```python
from build123d import *

# Parameters (mm, degrees)
SKETCH1_R           = 2
BOSS_EXTRUDE1_DEPTH = 89
SKETCH2_R           = 3
BOSS_EXTRUDE2_DEPTH = 2
CHAMFER1_SIZE       = 1


with BuildPart() as part:
    # Sketch1 → Boss-Extrude1 (new body)
    with BuildSketch(Plane(origin=(0, 0, 0), x_dir=(1, 0, 0), z_dir=(0, 1, 0))):
        with Locations(Location((0, 0, 0), (0, 0, 270))):
            Circle(SKETCH1_R)
    extrude(amount=BOSS_EXTRUDE1_DEPTH)

    # Sketch2 → Boss-Extrude2 (add)
    with BuildSketch(Plane.XZ):
        with Locations(Location((0, 0, 0), (0, 0, 270))):
            Circle(SKETCH2_R)
    extrude(amount=BOSS_EXTRUDE2_DEPTH)

    # Chamfer1
    chamfer1_edges = [part.edges().sort_by_distance(p)[0] for p in [
        (0, -2, 3),
    ]]
    chamfer(chamfer1_edges, length=CHAMFER1_SIZE)


solid = part.part
```
Check sheet for the modelled part. Datum: model origin and axes. Units: mm. A direction names the side the tool comes from. Give positions to 0.01 mm unless a question says otherwise; leave off trailing zeros. Write each loop counter-clockwise with the first axis right and the second up, starting at its lowest first coordinate (ties: lowest second). Pieces come first, ordered by that corner, then holes.
Item 1: Scan lines: L1, parallel to Z at x = 0.2, y = 62.5; L2, parallel to X at y = 50, z = 0; L3, parallel to Z at x = 0.65, y = 81. Record each from-to range of solid material in increasing order.
Item 2: Gauge pin test, flat ends, axial feed: pin 1 (2 mm diameter, centred on x = 2, y = 35, fed in from -Z); pin 2 (3 mm diameter, centred on y = 29.5, z = 0, fed in from +X). Record the tip position at first contact, or that the pin passes through.
Item 3: Access from +Z, -Z, +X, -X, +Y, -Y to the whole of each face (thin tool, end or side, straight path). Record for faces 1 (the face through (-1, 0, -2)), 2 (the face through (0, 89, 0)).
Item 4: Cross-section at B-B (z = 0). Enter the section's corners in (x, y).
Item 5: Cross-section at C-C (y = 78). Enter the section's corners in (x, z).
Item 6: Cross-section at A-A (x = 0). Enter the section's corners in (y, z), and give its area (3 significant figures).
Report:
1. L1: z = -1.99 to 1.99
1. L2: x = -2 to 2
1. L3: z = -1.89 to 1.89
2. pin 1: stops at z = -1.73
2. pin 2: stops at x = 2
3. face 1: +Y
3. face 2: +Z, -Z, +X, -X, +Y
4. outline: (-3, -1) - (-2, -2) - (2, -2) - (3, -1) - (3, 0) - (2, 0) - (2, 89) - (-2, 89) - (-2, 0) - (-3, 0) - close
5. outline: circle Ø4 at (0, 0)
6. outline: (-2, -2) - (-1, -3) - (0, -3) - (0, -2) - (89, -2) - (89, 2) - (0, 2) - (0, 3) - (-1, 3) - (-2, 2) - close
6. area: 367 mm2
